Work out the finished part from the listing and answer in its coordinate system (mm). Face numbers are marked on the shaded views. A direction names the side the tool comes from. Give positions to 0.01 mm unless a question says otherwise; leave off trailing zeros. Loops run counter-clockwise (first coordinate to the right, second up) from the corner with the lowest first, then second, coordinate; pieces in that order, holes last.
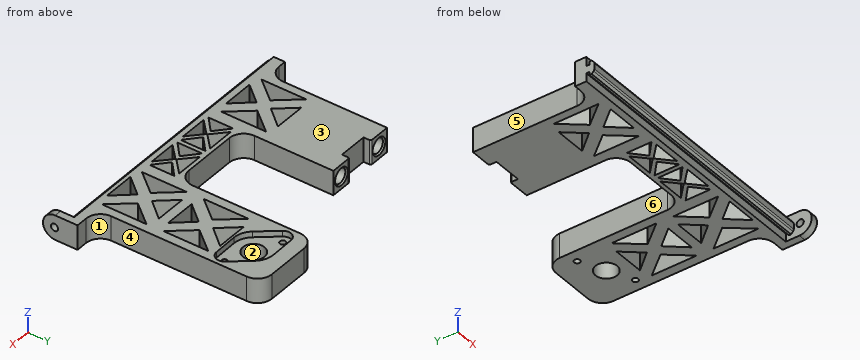
```python
from build123d import *

# Parameters (mm, degrees)
CROQUIS1_R              = 7.5
SALIENTE_EXTRUIR1_DEPTH = 17
REDONDEO1_R             = 10
REDONDEO2_R             = 10
REDONDEO8_R             = 10
REDONDEO9_R             = 10
REDONDEO11_R            = 10
REDONDEO12_R            = 10
SALIENTE_EXTRUIR2_DEPTH = 186
CROQUIS5_R              = 2.5
SALIENTE_EXTRUIR6_DEPTH = 5
CORTAR_EXTRUIR5_DEPTH   = 4
SKETCH3_R               = 2
CUT_EXTRUDE1_DEPTH      = 156.476686355
SKETCH4_R               = 5
CUT_EXTRUDE2_DEPTH      = 17.5
FILLET1_R               = 1
CHAMFER1_SIZE           = 1


with BuildPart() as part:
    # Croquis1 → Saliente-Extruir1 (new body)
    with BuildSketch(Plane.XY):
        Polygon((-93, 0), (93, 0), (93, 6), (80, 6), (80, 120), (30, 120), (30, 25.267194249), (-27.720969348, 25.267194249), (-27.720969348, 90), (-42.720969348, 90), (-42.720969348, 84.845258293), (-62.720969348, 84.845258293), (-62.720969348, 90), (-77.720969348, 90), (-77.720969348, 7.786589187), (-93, 7.786589187), align=None)
        Polygon((-53.370368055, 17.608830496), (-42.369998576, 4.626570416), (-64.231453048, 4.626570416), align=None, mode=Mode.SUBTRACT)
        Polygon((-72.099249791, 38.14298816), (-59.370368055, 22.608830496), (-72.099249791, 7.074672833), align=None, mode=Mode.SUBTRACT)
        Polygon((-3.458697993, 3.711831174), (-22.689998763, 3.711831174), (-13.074348378, 12.870825965), align=None, mode=Mode.SUBTRACT)
        Polygon((-26.085940215, 4.558933089), (-26.085940215, 21.785882097), (-16.561331103, 13.172407593), align=None, mode=Mode.SUBTRACT)
        Polygon((-9.587365653, 13.172407593), (-0.062756541, 21.785882097), (-0.062756541, 4.558933089), align=None, mode=Mode.SUBTRACT)
        Polygon((-34.641486319, 7.074672833), (-47.370368055, 22.608830496), (-34.641486319, 38.14298816), align=None, mode=Mode.SUBTRACT)
        Polygon((-13.074348378, 13.411373354), (-22.689998763, 22.570368145), (-3.458697993, 22.570368145), align=None, mode=Mode.SUBTRACT)
        Polygon((-53.370368055, 27.608830496), (-64.231453048, 40.591090577), (-42.369998576, 40.591090577), align=None, mode=Mode.SUBTRACT)
        Polygon((2.908210147, 4.558933089), (2.908210147, 21.785882097), (12.432819259, 13.172407593), align=None, mode=Mode.SUBTRACT)
        Polygon((6.304151599, 3.711831174), (15.919801984, 12.870825965), (25.535452369, 3.711831174), align=None, mode=Mode.SUBTRACT)
        Polygon((28.931393821, 21.785882097), (28.931393821, 4.558933089), (19.406784708, 13.172407593), align=None, mode=Mode.SUBTRACT)
        Polygon((6.304151599, 22.632984011), (25.535452369, 22.632984011), (15.919801984, 13.47398922), align=None, mode=Mode.SUBTRACT)
        Polygon((36.750632631, 36.163668304), (49.479514367, 20.629510641), (36.750632631, 5.095352977), align=None, mode=Mode.SUBTRACT)
        Polygon((55, 15.629510641), (66.000369479, 2.64725056), (44.138915007, 2.64725056), align=None, mode=Mode.SUBTRACT)
        Polygon((74.208396103, 5.095352977), (61.479514367, 20.629510641), (74.208396103, 36.163668304), align=None, mode=Mode.SUBTRACT)
        Polygon((55, 25.629510641), (44.138915007, 38.611770721), (66.000369479, 38.611770721), align=None, mode=Mode.SUBTRACT)
        Polygon((55, 58.101191757), (66.000369479, 45.118931676), (44.138915007, 45.118931676), align=None, mode=Mode.SUBTRACT)
        Polygon((36.271118264, 78.63534942), (49, 63.101191757), (36.271118264, 47.567034093), align=None, mode=Mode.SUBTRACT)
        Polygon((73.728881736, 47.567034093), (61, 63.101191757), (73.728881736, 78.63534942), align=None, mode=Mode.SUBTRACT)
        Polygon((55, 68.101191757), (44.138915007, 81.083451837), (66.000369479, 81.083451837), align=None, mode=Mode.SUBTRACT)
        with Locations((55, 96.25)):
            Circle(CROQUIS1_R, mode=Mode.SUBTRACT)
    extrude(amount=SALIENTE_EXTRUIR1_DEPTH)

    # Redondeo1
    redondeo1_edges = [part.edges().sort_by_distance(p)[0] for p in [
        (80, 120, 8.5),
    ]]
    fillet(redondeo1_edges, radius=REDONDEO1_R)

    # Redondeo2
    redondeo2_edges = [part.edges().sort_by_distance(p)[0] for p in [
        (30, 120, 8.5),
    ]]
    fillet(redondeo2_edges, radius=REDONDEO2_R)

    # Redondeo8
    redondeo8_edges = [part.edges().sort_by_distance(p)[0] for p in [
        (30, 25.267194249, 8.5),
    ]]
    fillet(redondeo8_edges, radius=REDONDEO8_R)

    # Redondeo9
    redondeo9_edges = [part.edges().sort_by_distance(p)[0] for p in [
        (-27.720969348, 25.267194249, 8.5),
    ]]
    fillet(redondeo9_edges, radius=REDONDEO9_R)

    # Redondeo11
    redondeo11_edges = [part.edges().sort_by_distance(p)[0] for p in [
        (80, 6, 8.5),
    ]]
    fillet(redondeo11_edges, radius=REDONDEO11_R)

    # Redondeo12
    redondeo12_edges = [part.edges().sort_by_distance(p)[0] for p in [
        (-77.720969348, 7.786589187, 8.5),
    ]]
    fillet(redondeo12_edges, radius=REDONDEO12_R)

    # Croquis4 → Saliente-Extruir2 (add)
    with BuildSketch(Plane.ZY.offset(93)):
        with BuildLine():
            Line((5.614135824, 0), (5.614135824, -2.2))
            Line((5.614135824, -2.2), (3.414135824, -2.2))
            Line((3.414135824, -2.2), (3.414135824, -3.7))
            Line((3.414135824, -3.7), (4.862457658, -5.028042266))
            ThreePointArc((4.862457658, -5.028042266), (5.488945101, -5.4178372), (6.214135824, -5.553943851))
            Line((6.214135824, -5.553943851), (10.014135824, -5.553943851))
            ThreePointArc((10.014135824, -5.553943851), (10.739326546, -5.4178372), (11.365813989, -5.028042266))
            Line((11.365813989, -5.028042266), (12.814135824, -3.7))
            Line((12.814135824, -3.7), (12.814135824, -2.2))
            Line((12.814135824, -2.2), (10.614135824, -2.2))
            Line((10.614135824, -2.2), (10.614135824, 0))
            Line((10.614135824, 0), (5.614135824, 0))
        make_face()
    extrude(amount=-SALIENTE_EXTRUIR2_DEPTH)

    # Croquis5 → Saliente-Extruir6 (add)
    with BuildSketch(Plane(origin=(93, 0, 0), x_dir=(0, 0, -1), z_dir=(1, 0, 0))):
        with BuildLine():
            Line((-17, 6), (0, 6))
            Line((0, 6), (0, 0))
            Line((0, 0), (0, -9.475176398))
            ThreePointArc((0, -9.475176398), (-8.5, -17.975176398), (-17, -9.475176398))
            Line((-17, -9.475176398), (-17, 0))
            Line((-17, 0), (-17, 6))
        make_face()
        with Locations(Location((-8.5, -10, 0), (0, 0, 90))):
            Circle(CROQUIS5_R, mode=Mode.SUBTRACT)
    extrude(amount=SALIENTE_EXTRUIR6_DEPTH)

    # Croquis13 → Cortar-Extruir5 (cut)
    with BuildSketch(Plane.XY.offset(17)):
        with BuildLine():
            Line((71.768371079, 82.874584815), (55.225000256, 82.601854526))
            ThreePointArc((55.225000256, 82.601854526), (49.231260727, 83.878898707), (44.400286624, 87.649501389))
            Line((44.400286624, 87.649501389), (33.975336359, 100.49776633))
            ThreePointArc((33.975336359, 100.49776633), (33.248613111, 106.392838282), (38.231628921, 109.625415185))
            Line((38.231628921, 109.625415185), (54.774999744, 109.898145474))
            ThreePointArc((54.774999744, 109.898145474), (60.768739273, 108.621101293), (65.599713376, 104.850498611))
            Line((65.599713376, 104.850498611), (76.024663641, 92.00223367))
            ThreePointArc((76.024663641, 92.00223367), (76.751386889, 86.107161718), (71.768371079, 82.874584815))
        make_face()
    extrude(amount=-CORTAR_EXTRUIR5_DEPTH, mode=Mode.SUBTRACT)

    # Sketch3 → Cut-Extrude1 (cut, through all)
    with BuildSketch(Plane.XY.offset(13)):
        with Locations((38.323936719, 104.02617602)):
            Circle(SKETCH3_R)
        with Locations((71.676063281, 88.47382398)):
            Circle(SKETCH3_R)
    extrude(amount=-CUT_EXTRUDE1_DEPTH, mode=Mode.SUBTRACT)

    # Sketch4 → Cut-Extrude2 (cut)
    with BuildSketch(Plane(origin=(0, 90, 0), x_dir=(1, 0, 0), z_dir=(0, 1, 0))):
        with Locations(Location((-70.220969348, -8.5, 0), (0, 0, 270))):
            Circle(SKETCH4_R)
        with Locations(Location((-35.220969348, -8.5, 0), (0, 0, 270))):
            Circle(SKETCH4_R)
    extrude(amount=-CUT_EXTRUDE2_DEPTH, mode=Mode.SUBTRACT)

    # Fillet1
    fillet1_edges = [part.edges().sort_by_distance(p)[0] for p in [
        (-62.720969348, 90, 8.5),
        (-42.720969348, 90, 8.5),
    ]]
    fillet(fillet1_edges, radius=FILLET1_R)

    # Chamfer1
    chamfer1_edges = [part.edges().sort_by_distance(p)[0] for p in [
        (-70.220969348, 90, 3.5),
        (-35.220969348, 90, 3.5),
    ]]
    chamfer(chamfer1_edges, length=CHAMFER1_SIZE)


solid = part.part
```
Q1. Consider line 1 along Y through (x, z) = (55, 7.5); line 2 along X through (y, z) = (46, 12.25); line 3 along X through (y, z) = (25, 15.5). Determine where each line is inside the solid, lowest interval first.
Q2. Determine the mould class of the marked faces 1, 2 and 3 for opening direction Y: +Y half, -Y half, draft (parallel to the pull), parting line (faces both ways), or undercut.
Q3. Section A-A on y = 96.25 is taken. Give the vertices of the cut face in (x, z), plus the area to 3 significant figures.
Q4. Which of the six approach directions +Z, -Z, +X, -X, +Y, -Y give full straight-line access (tool end or side, diameter ignored) to the marked faces 4, 5 and 6?
Q5. Given pin 1 (4 mm diameter, centred on x = -70.5, z = 12, fed in from -Y); pin 2 (10 mm diameter, centred on x = 52.5, y = 39, fed in from -Z); pin 3 (8.5 mm diameter, centred on y = 56, z = 7.5, fed in from -X); pin 4 (1.5 mm diameter, centred on x = 33, z = 4.5, fed in from +Y), each flat-ended and moving along its own axis, determine where each tip first touches the part or whether it passes through.
Check result:
1. line 1: y = -5.55 to 2.65, 15.63 to 25.63, 38.61 to 45.12, 58.1 to 68.1, 81.08 to 88.75, 103.75 to 120
1. line 2: x = -77.72 to -27.72, 30 to 44.88, 65.25 to 80
1. line 3: x = -77.72 to -72.1, -61.33 to -45.41, -34.64 to 36.75, 45.9 to 65.06, 74.21 to 80
2. face 1: +Y half
2. face 2: undercut
2. face 3: draft
3. outline: (30, 0) - (47.5, 0) - (47.5, 13) - (37.42, 13) - (37.42, 17) - (30, 17) - close; (62.5, 0) - (80, 0) - (80, 17) - (72.58, 17) - (72.58, 13) - (62.5, 13) - close
3. area: 514 mm2
4. face 4: +Z, -Z, +X, +Y
4. face 5: +Z, -Z, -X, +Y
4. face 6: +Z, -Z, +Y
5. pin 1: stops at y = -5.55
5. pin 2: stops at z = 0
5. pin 3: stops at x = -77.72
5. pin 4: stops at y = 117.81
